from build123d import *

# Parameters (mm, degrees)
SKETCH_1_R          = 1.625
EXTRUDE_1_DEPTH     = 3
FILLET_1_R          = 10
SKETCH_2_R          = 1.75
CUT_EXTRUDE_1_DEPTH = 10
SKETCH_4_R          = 1.75
CUT_EXTRUDE_2_DEPTH = 10
SKETCH_5_R          = 1.75
CUT_EXTRUDE_3_DEPTH = 10
CUT_EXTRUDE_4_DEPTH = 10
FILLET_2_R          = 3


with BuildPart() as part:
    # Эскиз1 → Бобышка-Вытянуть1 (new body)
    with BuildSketch(Plane.XY):
        with BuildLine():
            ThreePointArc((-32.5, -28.5), (-35.328427125, -35.328427125), (-28.5, -32.5))
            Line((-28.5, -32.5), (28.5, -32.5))
            ThreePointArc((28.5, -32.5), (35.328427125, -35.328427125), (32.5, -28.5))
            Line((32.5, -28.5), (32.5, 28.5))
            ThreePointArc((32.5, 28.5), (35.328427125, 35.328427125), (28.5, 32.5))
            Line((28.5, 32.5), (-28.5, 32.5))
            ThreePointArc((-28.5, 32.5), (-35.328427125, 35.328427125), (-32.5, 28.5))
            Line((-32.5, 28.5), (-32.5, -28.5))
        make_face()
        with Locations((-32.5, -32.5)):
            Circle(SKETCH_1_R, mode=Mode.SUBTRACT)
        with Locations((32.5, 32.5)):
            Circle(SKETCH_1_R, mode=Mode.SUBTRACT)
        with Locations((-32.5, 32.5)):
            Circle(SKETCH_1_R, mode=Mode.SUBTRACT)
        with Locations((32.5, -32.5)):
            Circle(SKETCH_1_R, mode=Mode.SUBTRACT)
    extrude(amount=EXTRUDE_1_DEPTH)

    # Скругление1
    fillet_1_edges = [part.edges().sort_by_distance(p)[0] for p in [
        (-32.5, -28.5, 1.5),
        (-32.5, 28.5, 1.5),
        (-28.5, 32.5, 1.5),
        (28.5, 32.5, 1.5),
        (32.5, 28.5, 1.5),
        (32.5, -28.5, 1.5),
        (28.5, -32.5, 1.5),
        (-28.5, -32.5, 1.5),
    ]]
    fillet(fillet_1_edges, radius=FILLET_1_R)

    # Эскиз2 → Вырез-Вытянуть1 (cut)
    with BuildSketch(Plane.XY.offset(3)):
        with Locations((-13, -25)):
            Circle(SKETCH_2_R)
        with Locations((13, -25)):
            Circle(SKETCH_2_R)
    extrude(amount=-CUT_EXTRUDE_1_DEPTH, mode=Mode.SUBTRACT)

    # Эскиз4 → Вырез-Вытянуть2 (cut)
    with BuildSketch(Plane.XY.offset(3)):
        with Locations((-16.5, -15)):
            Circle(SKETCH_4_R)
        with Locations((16.5, -15)):
            Circle(SKETCH_4_R)
    extrude(amount=-CUT_EXTRUDE_2_DEPTH, mode=Mode.SUBTRACT)

    # Эскиз5 → Вырез-Вытянуть3 (cut)
    with BuildSketch(Plane.XY.offset(3)):
        with Locations((-16.5, 5)):
            Circle(SKETCH_5_R)
        with Locations((16.5, 5)):
            Circle(SKETCH_5_R)
    extrude(amount=-CUT_EXTRUDE_3_DEPTH, mode=Mode.SUBTRACT)

    # Эскиз7 → Вырез-Вытянуть4 (cut)
    with BuildSketch(Plane.XY.offset(3)):
        Polygon((-24.5, 25), (24.5, 25), (27.5, 22), (27.5, 13), (24.5, 10), (-24.5, 10), (-27.5, 13), (-27.5, 22), align=None)
    extrude(amount=-CUT_EXTRUDE_4_DEPTH, mode=Mode.SUBTRACT)

    # Скругление2
    fillet_2_edges = [part.edges().sort_by_distance(p)[0] for p in [
        (-27.5, 22, 1.5),
        (-24.5, 25, 1.5),
        (24.5, 25, 1.5),
        (27.5, 22, 1.5),
        (27.5, 13, 1.5),
        (24.5, 10, 1.5),
        (-24.5, 10, 1.5),
        (-27.5, 13, 1.5),
    ]]
    fillet(fillet_2_edges, radius=FILLET_2_R)


solid = part.part
Can you work these out from the model? Positions are in its coordinate system, mm. A direction names the side the tool comes from. Give positions to 0.01 mm unless a question says otherwise; leave off trailing zeros. Order: outer loops, then holes, each group sorted by start corner. A loop starts at its lowest first (then second) coordinate and runs counter-clockwise, first axis right, second up. Notation, with made-up numbers: M 75.5,7.5 L 130.5,7.5 A23 ccw 130.5,32.5 Z; hole C -37,79 d2. An arc over 180 degrees is marked long. Use one line per item in the form item = value. Start each with the question number.
Item 1: Will these pins go through, and if not, where does the flat tip stop? pin 1 Ø2 at (x, y) = (-16.5, 5) entering from +Z; pin 2 Ø0.9 at (y, z) = (16.5, 2) entering from +X; pin 3 Ø1.5 at (y, z) = (16.5, 2) entering from -X; pin 4 Ø0.9 at (x, z) = (-4.5, 2) entering from -Y.
Item 2: If I drill on line 1 along Y through (x, z) = (16.5, 1.3); line 2 along Y through (x, z) = (13, 1.35); line 3 along X through (y, z) = (18, 1.4), over which ranges is the centre line in solid material (lowest first)?
Item 3: If we section it at A-A (x = -21.5): Write out the boundary of the cut face in (y, z), then the cut area to 3 significant figures.
Item 4: For faces 1 (the flat face through (-27.5, 17, 2)), 2 (the cylindrical face through (33.22, 26.43, 1.52)), 3 (the flat face through (8, -8, 0)), 4 (the cylindrical face through (26.43, -33.22, 1.52)), 5 (the flat face through (-32.5, 0, 1)), which set-ups out of +Z, -Z, +X, -X, +Y, -Y let a thin tool reach every point of the face, with its end or its side?
Item 5: If we section it at D-D (z = 1.85): State how many separate pieces and enclosed holes the cut face has, then the cut area to 3 significant figures.
Item 6: If we section it at B-B (y = -15): Write out the boundary of the cut face in (x, z).
Item 7: If we section it at C-C (x = 13): Write out the boundary of the cut face in (y, z), then the cut area to 4 significant figures.
Item 8: We'd pull the mould along Y, two halves only. Please class faces 6 (the flat face through (8, -8, 3)), 7 (the cylindrical face through (-26.53, -33.26, 1.52)), 8 (the cylindrical face through (35.266, -35.39, 1.479)): +Y half, -Y half, draft (parallel to the pull), parting line (faces both ways), or undercut.
Outcome:
q1.pin_1 = through
q1.pin_2 = 32.5
q1.pin_3 = -32.5
q1.pin_4 = -32.5
q2.line_1 = -32.5 to -16.75, -13.25 to 3.25, 6.75 to 10, 25 to 32.5
q2.line_2 = -32.5 to -26.75, -23.25 to 10, 25 to 32.5
q2.line_3 = -32.5 to -27.5, 27.5 to 32.5
q3.outline = M -32.5,0 L 10,0 L 10,3 L -32.5,3 Z; M 25,0 L 32.5,0 L 32.5,3 L 25,3 Z
q3.area = 150 mm2
q4.face_1 = +Z, -Z
q4.face_2 = +Z, -Z, +X
q4.face_3 = -Z, +X, -X, +Y, -Y
q4.face_4 = +Z, -Z, -Y
q4.face_5 = +Z, -Z, -X
q5.separate_pieces = 1
q5.enclosed_holes = 11
q5.area = 3,510 mm2
q6.outline = M -32.5,0 L -18.25,0 L -18.25,3 L -32.5,3 Z; M -14.75,0 L 14.75,0 L 14.75,3 L -14.75,3 Z; M 18.25,0 L 32.5,0 L 32.5,3 L 18.25,3 Z
q7.outline = M -32.5,0 L -26.75,0 L -26.75,3 L -32.5,3 Z; M -23.25,0 L 10,0 L 10,3 L -23.25,3 Z; M 25,0 L 32.5,0 L 32.5,3 L 25,3 Z
q7.area = 139.5 mm2
q8.face_6 = draft
q8.face_7 = -Y half
q8.face_8 = undercut
